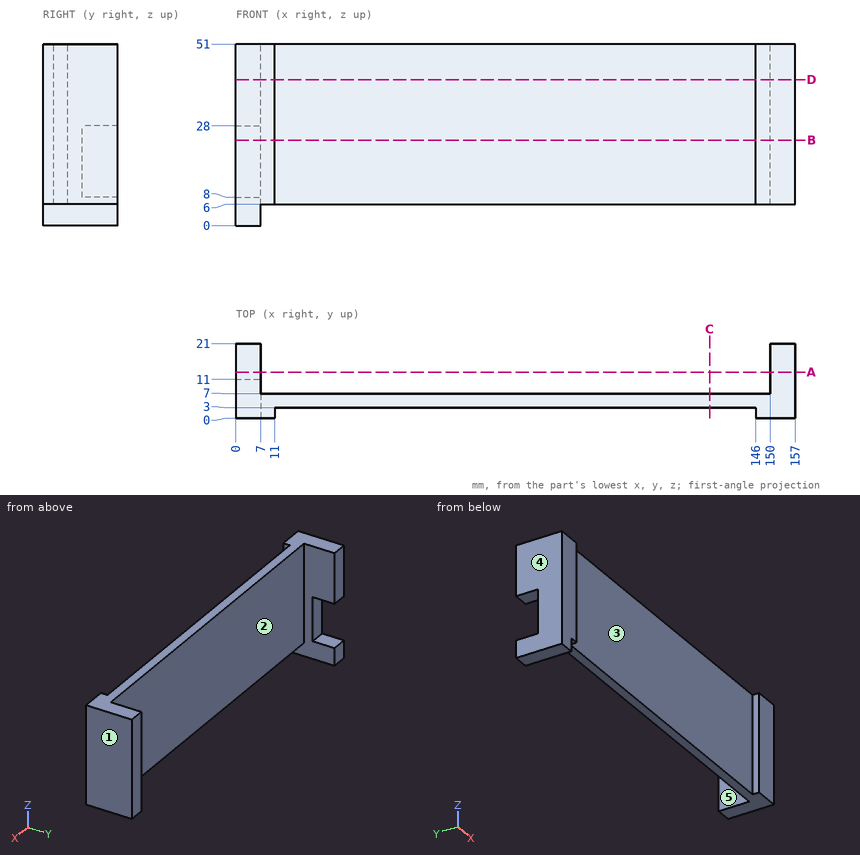
Part print with two shaded views. Sizes in mm from the minimum x, y, z corner. A direction names the side the tool comes from. Coordinates: 2 decimals unless noted, no trailing zeros. Loops run counter-clockwise (first coordinate to the right, second up) from the corner with the lowest first, then second, coordinate; pieces in that order, holes last. Notation, with made-up numbers: (61, 18) - (102, 18) arc R7 cw to (102, 26) - close; hole circle Ø6 at (-29.75, 74). An arc over 180 degrees is marked (long way). Write each question's results on one line, items separated by ' | '. Start each with the question number.
Q1. Which spindle directions (+Z, -Z, +X, -X, +Y, -Y) get a long thin tool onto all of the face, cutting with end or side? Do the marked faces 4 and 5. Say none if no direction does.
Q2. Probe line 1 along X through (y, z) = (2.5, 18.5); line 2 along X through (y, z) = (9.75, 28); line 3 along Y through (x, z) = (117, 43). List the from-to ranges inside material, lowest first.
Q3. Slice it at C-C on x = 133. Give the cut face in (y, z).
Q4. Slice it at A-A on y = 13. Give the cut face in (x, z), and give its area (3 significant figures).
Q5. Slice it at B-B on z = 24. Give the cut face in (x, y), and give its area (3 significant figures).
Q6. Drop flat-ended pins along their axis: pin 1 Ø13.5 at (x, z) = (106.5, 32) entering from +Y; pin 2 Ø8 at (x, y) = (137.5, 4) entering from -Z; pin 3 Ø12 at (x, z) = (90.5, 27.5) entering from -Y. Give the stop position or say it passes through.
Q7. Two-plate mould, pull along Y, no slides. Class the marked faces 1, 2 and 3: +Y half, -Y half, draft (parallel to the pull), parting line (faces both ways), or undercut.
Q8. Slice it at D-D on z = 41. Give the cut face in (x, y), and give its area (3 significant figures).
Answer:
1) face 4: +Z, -Z, -X, +Y, -Y | face 5: +Z, -Z, +Y
2) line 1: x = 0 to 11, 146 to 157 | line 2: x = 0 to 7, 150 to 157 | line 3: y = 3 to 7
3) outline: (3, 6) - (7, 6) - (7, 51) - (3, 51) - close
4) outline: (0, 0) - (7, 0) - (7, 8) - (0, 8) - close; (0, 28) - (7, 28) - (7, 51) - (0, 51) - close; (150, 6) - (157, 6) - (157, 51) - (150, 51) - close | area: 532 mm2
5) outline: (0, 0) - (11, 0) - (11, 3) - (146, 3) - (146, 0) - (157, 0) - (157, 21) - (150, 21) - (150, 7) - (7, 7) - (7, 11) - (0, 11) - close | area: 820 mm2
6) pin 1: stops at y = 7 | pin 2: stops at z = 6 | pin 3: stops at y = 3
7) face 1: draft | face 2: +Y half | face 3: -Y half
8) outline: (0, 0) - (11, 0) - (11, 3) - (146, 3) - (146, 0) - (157, 0) - (157, 21) - (150, 21) - (150, 7) - (7, 7) - (7, 21) - (0, 21) - close | area: 890 mm2
